Source: CAD feature listing. Evaluate the final solid. Frame: model axes, mm. A direction names the side the tool comes from. Give positions to 0.01 mm unless a question says otherwise; leave off trailing zeros. Return JSON: item names as keys, results as strings. Group by question number.
```python
from build123d import *

# Parameters (mm, degrees)
BOSS_EXTRUDE1_DEPTH = 110
BOSS_EXTRUDE2_DEPTH = 3
LPATTERN1_COUNT     = 15
LPATTERN1_PITCH     = 7


with BuildPart() as part:
    # Sketch1 → Boss-Extrude1 (new body)
    with BuildSketch(Plane(origin=(0, 0, 0), x_dir=(1, 0, 0), z_dir=(0, 1, 0))):
        with BuildLine():
            Line((63, 0), (78, 0))
            ThreePointArc((78, 0), (103, 25), (128, 0))
            Line((128, 0), (143, 0))
            ThreePointArc((143, 0), (168, 25), (193, 0))
            Line((193, 0), (208, 0))
            ThreePointArc((208, 0), (233, 25), (258, 0))
            Line((258, 0), (271, 0))
            Line((271, 0), (271, 55))
            ThreePointArc((271, 55), (268.071067812, 62.071067812), (261, 65))
            Line((261, 65), (10, 65))
            ThreePointArc((10, 65), (2.928932188, 62.071067812), (0, 55))
            Line((0, 55), (0, 0))
            Line((0, 0), (13, 0))
            ThreePointArc((13, 0), (38, 25), (63, 0))
        make_face()
    extrude(amount=BOSS_EXTRUDE1_DEPTH)

    # Sketch4 → Boss-Extrude2 (add)
    with BuildSketch(Plane.XZ):
        with BuildLine():
            Line((-4, 0), (-4, -55))
            ThreePointArc((-4, -55), (0.100505063, -64.899494937), (10, -69))
            Line((10, -69), (261, -69))
            ThreePointArc((261, -69), (270.899494937, -64.899494937), (275, -55))
            Line((275, -55), (275, 0))
            Line((275, 0), (271, 0))
            Line((271, 0), (271, -55))
            ThreePointArc((271, -55), (268.071067812, -62.071067812), (261, -65))
            Line((261, -65), (10, -65))
            ThreePointArc((10, -65), (2.928932188, -62.071067812), (0, -55))
            Line((0, -55), (0, 0))
            Line((0, 0), (-4, 0))
        make_face()
    boss_extrude2 = extrude(amount=-BOSS_EXTRUDE2_DEPTH)

    # LPattern1: Boss-Extrude2 ×15
    with Locations(*[(0, i * LPATTERN1_PITCH, 0) for i in range(1, LPATTERN1_COUNT)]):
        add(boss_extrude2)


solid = part.part
```
1) Cut plane A-A on z = -20. Count the separate pieces of the cut face and the enclosed holes in it, then the cut area to 3 significant figures.
2) Reachability of faces 1 (the face through (3.01, 67.97, -62.15)), 2 (the face through (268.15, 53.97, -61.99)), 3 (the face through (0, 15.5, -64.8)) from +Z, -Z, +X, -X, +Y, -Y: full face, straight path, thin tool, end or side. Return the list, or none.
3) Mould query, pull axis Y, two halves, no side actions, for faces 4 (the face through (0, 64.5, -64.8)), 5 (the face through (268.15, 67.97, -61.99)), 6 (the face through (135, 101, -68)). Classes: released by +Y, released by -Y, zero draft, split by the parting line, or undercut.
4) Contact query for flat-ended pins moving along their axis: P1, Ø2, axis at x = 201, y = 25.5, coming from the -Z side; P2, Ø8, axis at x = 244.5, y = 92, coming from the +Z side; P3, Ø4, axis at x = 106, y = 62.5, coming from the +Z side. Output: stop coordinate, or through.
5) Material intervals for line 1 (X direction, y = 8, z = -9); line 2 (X direction, y = 45.5, z = -29); line 3 (Z direction, x = 141.5, y = 47), sorted ascending.
Calculated:
{
 "1": {"separate pieces": "5", "enclosed holes": "0", "area": "17,000 mm2"},
 "2": {"face 1": "-Z, -X", "face 2": "-Z, +X", "face 3": "-Z, -X, +Y, -Y"},
 "3": {"face 4": "zero draft", "face 5": "undercut", "face 6": "released by +Y"},
 "4": {"P1": "z = -65", "P2": "z = -19.62", "P3": "z = -24.49"},
 "5": {"line 1": "-4 to 14.68, 61.32 to 79.68, 126.32 to 144.68, 191.32 to 209.68, 256.32 to 275", "line 2": "0 to 271", "line 3": "-65 to 0"}
}
